Read the model definition and answer for the solid it produces. Units are mm, in the model's axes. A direction names the side the tool comes from. Give positions to 0.01 mm unless a question says otherwise; leave off trailing zeros. Write each loop counter-clockwise with the first axis right and the second up, starting at its lowest first coordinate (ties: lowest second). Pieces come first, ordered by that corner, then holes. Notation, with made-up numbers: (2, 4) -> (32, 4) arc R26 cw to (32, 29) -> close; hole circle Ø10 at (22.5, 52). An arc over 180 degrees is marked (long way). Write item = value, one per line.
from build123d import *

# Parameters (mm, degrees)
SKETCH_R     = 7
PAD_DEPTH    = 10
SKETCH001_R  = 2.5
POCKET_DEPTH = 39.001
PAD001_DEPTH = 3
FILLET_R     = 1


with BuildPart() as pocket:
    # Sketch → Pad (new body, symmetric)
    with BuildSketch(Plane.XZ):
        with BuildLine():
            ThreePointArc((1.5, -15.929532), (0, 16), (-1.5, -15.929532))
            Line((-1.5, -32.734994), (-1.5, -15.929532))
            Line((-1.5, -32.734994), (-15, -32.734994))
            Line((-15, -32.734994), (-15, -18.734994))
            ThreePointArc((23.811762, 3), (-11.726648, 20.940051), (-15, -18.734994))
            Line((23.811762, 3), (42.350889, 3))
            ThreePointArc((42.350889, -3), (68, 0), (42.350889, 3))
            Line((42.350889, -3), (23.811762, -3))
            ThreePointArc((15, -18.734994), (20.940051, -11.726648), (23.811762, -3))
            Line((15, -18.734994), (15, -32.734994))
            Line((15, -32.734994), (1.5, -32.734994))
            Line((1.5, -15.929532), (1.5, -32.734994))
        make_face()
        with Locations((55, 0)):
            Circle(SKETCH_R, mode=Mode.SUBTRACT)
    extrude(amount=PAD_DEPTH, both=True)

    # Sketch001 → Pocket (cut, through all)
    with BuildSketch(Plane(origin=(15, 0, 0), x_dir=(0, 0, 1), z_dir=(1, 0, 0))):
        with Locations((-25.734994, 0)):
            Circle(SKETCH001_R)
    extrude(amount=-POCKET_DEPTH, mode=Mode.SUBTRACT)


with BuildPart() as fillet_body:
    # Sketch002 → Pad001 (new body, symmetric)
    with BuildSketch(Plane.XZ):
        with BuildLine():
            Line((23.811762, 3), (42.350889, 3))
            ThreePointArc((55, 13), (46.937742, 10.198039), (42.350889, 3))
            Line((20.174241, 13), (55, 13))
            ThreePointArc((23.811762, 3), (22.554204, 8.204139), (20.174241, 13))
        make_face()
    extrude(amount=PAD001_DEPTH, both=True)

    # Fusion: union Pocket
    add(pocket.part)

    # Fillet
    fillet_edges = [fillet_body.edges().sort_by_distance(p)[0] for p in [
        (20.174241, 0, 13),
    ]]
    fillet(fillet_edges, radius=FILLET_R)


solid = fillet_body.part
(1) The part is cut by section B-B on z = 0. Determine the outline of the cut face in (x, y).
Checks:
outline = (-24, -10) -> (-16, -10) -> (-16, 10) -> (-24, 10) -> close; (16, -10) -> (48, -10) -> (48, 10) -> (16, 10) -> close; (62, -10) -> (68, -10) -> (68, 10) -> (62, 10) -> close
(2) The part is cut by section A-A on y = 0. Determine the outline of the cut face in (x, z) (3 decimals).
Checks:
outline = (-15, -32.735) -> (-1.5, -32.735) -> (-1.5, -28.235) -> (-15, -28.235) -> close; (-15, -23.235) -> (-1.5, -23.235) -> (-1.5, -15.93) arc R16 cw (long way) to (1.5, -15.93) -> (1.5, -23.235) -> (15, -23.235) -> (15, -18.735) arc R24 ccw to (23.812, -3) -> (42.351, -3) arc R13 ccw (long way) to (55, 13) -> (20.712, 13) arc R1 cw to (19.884, 13.44) arc R24 ccw (long way) to (-15, -18.735) -> close; (1.5, -32.735) -> (15, -32.735) -> (15, -28.235) -> (1.5, -28.235) -> close; hole circle Ø14 at (55, 0)
(3) Given P1, Ø1.5, axis at x = 29, y = 3, coming from the +Z side; P2, Ø1.5, axis at y = -3.5, z = -20.5, coming from the +X side; P3, Ø4, axis at y = 0, z = -25.73, coming from the +X side; P4, Ø9.5, axis at x = 32.5, y = -0.5, coming from the -Z side, each flat-ended and moving along its own axis, determine where each tip first touches the part or whether it passes through.
Checks:
P1 = 13
P2 = 15
P3 = through
P4 = -3
(4) A tool of negligible diameter and unlimited length cuts with its end or side. For faces 1 (the flat face through (15, 2.1, -24.1)), 2 (the flat face through (33, 3, 9)), 3 (the flat face through (-1.5, 0, -23)), 4 (the cylindrical face through (8.344, 0.958, -23.426)), 5 (the flat face through (33, -3, 9)), from which of +Z, -Z, +X, -X, +Y, -Y can it reach the whole face along a straight path? Write none if from no direction.
Checks:
face_1 = -Z, +X, +Y, -Y
face_2 = +Z, +Y
face_3 = -Z, +Y, -Y
face_4 = +X, -X
face_5 = +Z, -Y
(5) The part is cut by section C-C on z = -22. Determine the outline of the cut face in (x, y).
Checks:
outline = (-15, -10) -> (-1.5, -10) -> (-1.5, 10) -> (-15, 10) -> close; (1.5, -10) -> (15, -10) -> (15, 10) -> (1.5, 10) -> close
(6) For a pull along X with two mould halves and no side action, classify faces 6 (the flat face through (-15, -2.4, -24.3)), 7 (the flat face through (33, -7, 3)), 8 (the cylindrical face through (61.677, 0.14, 2.103)), 9 (the flat face through (38, 0, 13)) as released by +X, released by -X, zero draft, split by the parting line, or undercut.
Checks:
face_6 = released by -X
face_7 = undercut
face_8 = undercut
face_9 = zero draft
(7) Consider L1, parallel to X at y = -4.25, z = -5.5; L2, parallel to Z at x = 55, y = 0.5; L3, parallel to Z at x = -5.5, y = 0 (3 decimals). Determine where each line is inside the solid, lowest interval first.
Checks:
L1 = -23.36 to -15.02, 15.02 to 23.36, 43.22 to 50.67, 59.33 to 66.78
L2 = -13 to -7, 7 to 13
L3 = -32.735 to -28.235, -23.235 to -15.025, 15.025 to 23.361
(8) The part is cut by section D-D on y = -4.75. Determine the outline of the cut face in (x, z) (3 decimals).
Checks:
outline = (-15, -32.735) -> (-1.5, -32.735) -> (-1.5, -15.93) arc R16 cw (long way) to (1.5, -15.93) -> (1.5, -32.735) -> (15, -32.735) -> (15, -18.735) arc R24 ccw to (23.812, -3) -> (42.351, -3) arc R13 ccw (long way) to (42.351, 3) -> (23.812, 3) arc R24 ccw (long way) to (-15, -18.735) -> close; hole circle Ø14 at (55, 0)
